Can you work these out from the model? Positions are in its coordinate system, mm. A direction names the side the tool comes from. Give positions to 0.01 mm unless a question says otherwise; leave off trailing zeros. Order: outer loops, then holes, each group sorted by start corner. A loop starts at its lowest first (then second) coordinate and runs counter-clockwise, first axis right, second up. Notation, with made-up numbers: M 4,-27 L 10,-27 A19 ccw 10,-12 Z; hole C 27.5,59 d10. An arc over 180 degrees is marked long. Answer as a JSON object with one key per item and string values.
Autodesk Inventor part; units mm, degrees
ref_plane "YZ Plane" through (0, 0, 0) normal (1, 0, 0) x (0, 1, 0)
ref_plane "XZ Plane" through (0, 0, 0) normal (0, 1, 0) x (-1, 0, 0)
ref_plane "XY Plane" through (0, 0, 0) normal (0, 0, 1) x (1, 0, 0)
sketch "Esquisse1" plane through (0, 0, 0) normal (0, 0, 1) x (1, 0, 0)
  circle A0 centre (0, 0) radius 9.5
  circle A1 centre (0, 0) radius 3
  dimension "d0" = 6
  dimension "d1" = 19
extrude "Extrusion1" add sketch "Esquisse1" along normal blind 6
fillet "Congé1" radius 1 2 edges at (-9.5, 0, 6) (-9.5, 0, 0)
sketch "Esquisse2" plane through (0, 0, 6) normal (0, 0, 1) x (1, 0, 0)
  circle A0 centre (0, 0) radius 4
  circle A1 centre (0, 0) radius 8.5
  dimension "d5" = 8
  dimension "d6" = 17
extrude "Extrusion2" cut sketch "Esquisse2" against normal blind 0.5
sketch "Esquisse3" plane through (0, 0, 0) normal (0, 0, -1) x (-1, 0, 0)
  circle A0 centre (0, 0) radius 4
  circle A1 centre (0, 0) radius 8.5
extrude "Extrusion3" cut sketch "Esquisse3" against normal blind 0.5
chamfer "Chanfrein3" distance 0.5 angle 45 2 edges at (-4, 0, 5.5) (-8.5, 0, 5.5)
chamfer "Chanfrein4" distance 0.5 angle 45 2 edges at (8.5, 0, 0.5) (4, 0, 0.5)
properties part number "Roulement"
1) I want a section at C-C on z = 2. Write out the boundary of the cut face in (x, y).
Results found:
{"outline": "C 0,0 d19; hole C 0,0 d6"}
2) I need wall thicknesses on L1, parallel to Z at x = 0, y = 5.5; L2, parallel to X at y = 1.5, z = 2.85; L3, parallel to Y at x = 2.25, z = 3.9. Which ranges of each line are inside material? Lowest first, please.
Results found:
{"L1": "z = 0.5 to 5.5", "L2": "x = -9.38 to -2.6, 2.6 to 9.38", "L3": "y = -9.23 to -1.98, 1.98 to 9.23"}
3) I'm going to push flat-ended pins straight in: pin 1 Ø3 at (x, z) = (4, 1.5) entering from -Y; pin 2 Ø2 at (x, y) = (5, -3) entering from -Z; pin 3 Ø3.5 at (x, y) = (0, 0) entering from -Z; pin 4 Ø2 at (y, z) = (-2, 4) entering from +X. Where does each tip first touch, or does it pass through?
Results found:
{"pin 1": "stops at y = -9.17", "pin 2": "stops at z = 0.5", "pin 3": "passes through", "pin 4": "stops at x = 9.45"}
4) Thinking about a two-plate mould opening in Y: for faces 1 (the face through (-3, 0, 3)), 2 (the face through (4.38, 8.43, 2.97)), 3 (the face through (-3.4, -3.4, 0.5)), 4 (the face through (1, 3, 6)), which applies, pulls with the +Y half, pulls with the -Y half, needs draft (parallel to the pull), parting line crosses it, or undercut?
Results found:
{"face 1": "undercut", "face 2": "parting line crosses it", "face 3": "undercut", "face 4": "needs draft"}
5) I want a section at D-D on z = 0.75. Write out the boundary of the cut face in (x, y), and give its area (3 significant figures).
Results found:
{"outline": "C 0,0 d18.94; hole C 0,0 d6", "area": "253 mm²"}
6) For faces 5 (the face through (3.4, -3.4, 5.5)), 6 (the face through (1, 3, 0)), which set-ups out of +Z, -Z, +X, -X, +Y, -Y let a thin tool reach every point of the face, with its end or its side?
Results found:
{"face 5": "+Z", "face 6": "-Z, +X, -X, +Y, -Y"}
